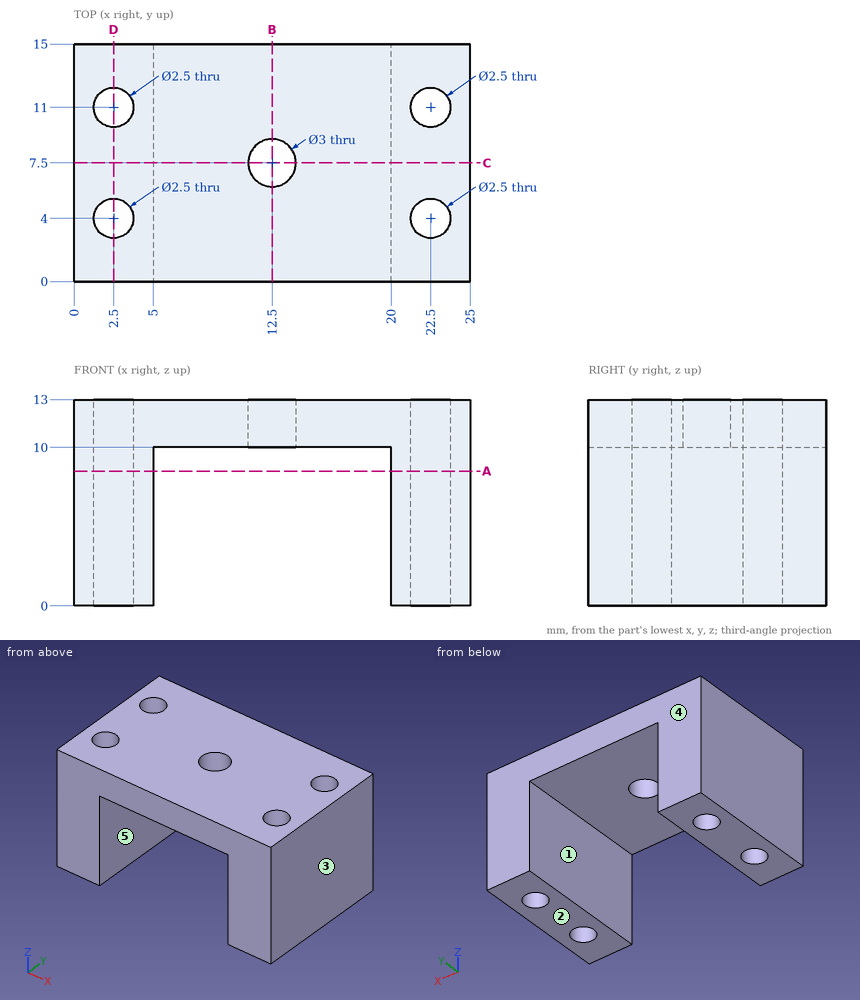
Source: three-view drawing plus pictorial views. Frame: mm from the lowest corner of the part. A direction names the side the tool comes from. Round coordinates to 2 decimals unless told otherwise and drop trailing zeros. Order: outer loops, then holes, each group sorted by start corner. A loop starts at its lowest first (then second) coordinate and runs counter-clockwise, first axis right, second up. Notation, with made-up numbers: (43.25, 58) - (58.25, 58) arc R27 ccw to (58.25, 89) - close; hole circle Ø5 at (52, 16). An arc over 180 degrees is marked (long way). Use a Markdown table: item, result.
1. First-contact query: pin 1 (4.5 mm diameter, centred on x = 11, y = 6, fed in from -Z). Flat tip, straight axial feed; report the tip coordinate or a pass-through.
Evaluation:
| item | result |
|---|---|
| pin 1 | z = 10 |
2. Access query for the marked faces 4 and 5. Directions: +Z, -Z, +X, -X, +Y, -Y. A direction counts if a zero-diameter tool reaches every point of the face in a straight line with its end or side. Return the directions, or none.
Evaluation:
| item | result |
|---|---|
| face 4 | +Z, -Z, +X, -X, +Y |
| face 5 | -Z, +Y, -Y |
3. Section B-B on x = 12.5. Return the cut outline in (y, z), then the cut area to 3 significant figures.
Evaluation:
| item | result |
|---|---|
| outline | (0, 10) - (6, 10) - (6, 13) - (0, 13) - close; (9, 10) - (15, 10) - (15, 13) - (9, 13) - close |
| area | 36.0 mm^2 |
4. Section C-C on y = 7.5. Return the cut outline in (x, z), then the cut area to 3 significant figures.
Evaluation:
| item | result |
|---|---|
| outline | (0, 0) - (5, 0) - (5, 10) - (11, 10) - (11, 13) - (0, 13) - close; (14, 10) - (20, 10) - (20, 0) - (25, 0) - (25, 13) - (14, 13) - close |
| area | 166 mm^2 |
5. Mould query, pull axis X, two halves, no side actions, for the marked faces 1, 2 and 3. Classes: +X half, -X half, draft (parallel to the pull), parting line (faces both ways), or undercut.
Evaluation:
| item | result |
|---|---|
| face 1 | undercut |
| face 2 | draft |
| face 3 | +X half |
6. Section A-A on z = 8.5. Return the cut outline in (x, y).
Evaluation:
| item | result |
|---|---|
| outline | (0, 0) - (5, 0) - (5, 15) - (0, 15) - close; (20, 0) - (25, 0) - (25, 15) - (20, 15) - close; hole circle Ø2.5 at (2.5, 4); hole circle Ø2.5 at (2.5, 11); hole circle Ø2.5 at (22.5, 4); hole circle Ø2.5 at (22.5, 11) |
7. Section D-D on x = 2.5. Return the cut outline in (y, z), then the cut area to 3 significant figures.
Evaluation:
| item | result |
|---|---|
| outline | (0, 0) - (2.75, 0) - (2.75, 13) - (0, 13) - close; (5.25, 0) - (9.75, 0) - (9.75, 13) - (5.25, 13) - close; (12.25, 0) - (15, 0) - (15, 13) - (12.25, 13) - close |
| area | 130 mm^2 |
8. Material intervals for probe 1 along Y at (x, z) = (2.5, 7.75); probe 2 along X at (y, z) = (7.5, 3.25); probe 3 along Z at (x, y) = (18, 1.25), sorted ascending.
Evaluation:
| item | result |
|---|---|
| probe 1 | 0 to 2.75, 5.25 to 9.75, 12.25 to 15 |
| probe 2 | 0 to 5, 20 to 25 |
| probe 3 | 10 to 13 |
